```python
from build123d import *

# Parameters (mm, degrees)
SKETCH1_R           = 2
SKETCH1_R_2         = 4.5
BOSS_EXTRUDE1_DEPTH = 10
SKETCH1_3_R         = 4.5
BOSS_EXTRUDE2_DEPTH = 10
CUT_EXTRUDE1_DEPTH  = 13
FILLET1_R           = 1
FILLET2_R           = 1
SKETCH3_R           = 2.5
CUT_EXTRUDE2_DEPTH  = 10


with BuildPart() as part:
    # Sketch1 → Boss-Extrude1 (new body)
    with BuildSketch(Plane(origin=(0, 0, 0), x_dir=(1, 0, 0), z_dir=(0, 1, 0))):
        with BuildLine():
            ThreePointArc((-12, 5), (-11.707106781, 5.707106781), (-11, 6))
            Line((-11, 6), (11, 6))
            ThreePointArc((11, 6), (11.707106781, 5.707106781), (12, 5))
            Line((12, 5), (12, -5))
            ThreePointArc((12, -5), (11.707106781, -5.707106781), (11, -6))
            Line((11, -6), (-11, -6))
            ThreePointArc((-11, -6), (-11.707106781, -5.707106781), (-12, -5))
            Line((-12, -5), (-12, 5))
        make_face()
        with Locations((-8, 0)):
            Circle(SKETCH1_R, mode=Mode.SUBTRACT)
        with Locations((8, 0)):
            Circle(SKETCH1_R, mode=Mode.SUBTRACT)
        Circle(SKETCH1_R_2, mode=Mode.SUBTRACT)
        Circle(SKETCH1_R_2)
    extrude(amount=BOSS_EXTRUDE1_DEPTH)

    # Sketch1_3 → Boss-Extrude2 (add)
    with BuildSketch(Plane(origin=(0, 0, 0), x_dir=(1, 0, 0), z_dir=(0, 1, 0))):
        Circle(SKETCH1_3_R)
    extrude(amount=-BOSS_EXTRUDE2_DEPTH)

    # Sketch2 → Cut-Extrude1 (cut, through all)
    with BuildSketch(Plane.XY.offset(6)):
        with BuildLine():
            Line((-5, 10), (5, 10))
            ThreePointArc((5, 10), (0, 5), (-5, 10))
        make_face()
    extrude(amount=-CUT_EXTRUDE1_DEPTH, mode=Mode.SUBTRACT)

    # Fillet1
    fillet1_edges = [part.edges().sort_by_distance(p)[0] for p in [
        (0, 0, -6),
        (11.707106781, 0, -5.707106781),
        (12, 0, 0),
        (11.707106781, 0, 5.707106781),
        (0, 0, 6),
        (-11.707106781, 0, 5.707106781),
        (-12, 0, 0),
        (-11.707106781, 0, -5.707106781),
        (-4.5, -10, 0),
    ]]
    fillet(fillet1_edges, radius=FILLET1_R)

    # Fillet2
    fillet2_edges = [part.edges().sort_by_distance(p)[0] for p in [
        (-4.5, 0, 0),
    ]]
    fillet(fillet2_edges, radius=FILLET2_R)

    # Sketch3 → Cut-Extrude2 (cut)
    with BuildSketch(Plane.XZ.offset(10)):
        Circle(SKETCH3_R)
    extrude(amount=-CUT_EXTRUDE2_DEPTH, mode=Mode.SUBTRACT)


solid = part.part
```
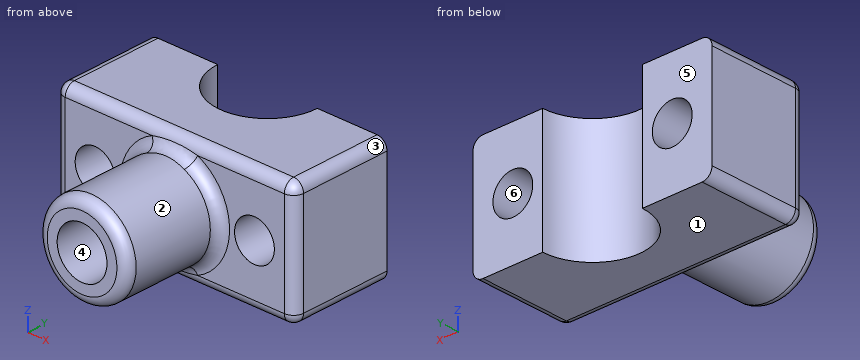
Geometry check sheet. Reference: the model listing, model coordinates, mm. Face numbers are marked on the shaded views. A direction names the side the tool comes from. Coordinates: 2 decimals unless noted, no trailing zeros. Loops run counter-clockwise (first coordinate to the right, second up) from the corner with the lowest first, then second, coordinate; pieces in that order, holes last.
Item 1: Sectioned sample at B-B, the plane y = 3.25. Record the boundary of the cut face in (x, z), then the cut area to 3 significant figures.
Item 2: Go/stop test with flat-tipped pins: pin 1 Ø2.5 at (x, z) = (-8, 0) entering from -Y; pin 2 Ø3 at (x, y) = (5.5, -4) entering from +Z; pin 3 Ø3 at (y, z) = (-4, -3.5) entering from +X; pin 4 Ø6 at (x, z) = (-6, 3) entering from -Y. Record where each tip stops, or that it passes through.
Item 3: Sectioned sample at C-C, the plane x = -8. Record the boundary of the cut face in (y, z).
Item 4: Access from +Z, -Z, +X, -X, +Y, -Y to the whole of each face (thin tool, end or side, straight path). Record for the marked faces 1 and 2.
Item 5: Sectioned sample at A-A, the plane y = 6. Record the boundary of the cut face in (x, z).
Item 6: Sectioned sample at D-D, the plane z = 0. Record the boundary of the cut face in (x, y).
Item 7: Release check for a two-part mould opening along Z. For the marked faces 3, 4, 5 and 6 record: released by +Z, released by -Z, zero draft, split by the parting line, or undercut.
Item 8: Thickness scan on line 1 (X direction, y = 2.25, z = 0); line 2 (Z direction, x = 8, y = 6.75); line 3 (X direction, y = 3, z = 1). Record the ranges inside material, lowest first.
Check result:
1. outline: (-12, -5) arc R1 ccw to (-11, -6) - (11, -6) arc R1 ccw to (12, -5) - (12, 5) arc R1 ccw to (11, 6) - (-11, 6) arc R1 ccw to (-12, 5) - close; hole circle Ø4 at (-8, 0); hole circle Ø4 at (8, 0)
1. area: 262 mm2
2. pin 1: passes through
2. pin 2: stops at z = 2.06
2. pin 3: stops at x = 4.03
2. pin 4: stops at y = -9.98
3. outline: (0, -5) arc R1 ccw to (1, -6) - (10, -6) - (10, -2) - (0, -2) - close; (0, 2) - (10, 2) - (10, 6) - (1, 6) arc R1 ccw to (0, 5) - close
4. face 1: -Z, +X, -X, +Y, -Y
4. face 2: -Y
5. outline: (-12, -5) arc R1 ccw to (-11, -6) - (-3, -6) - (-3, 6) - (-11, 6) arc R1 ccw to (-12, 5) - close; (3, -6) - (11, -6) arc R1 ccw to (12, -5) - (12, 5) arc R1 ccw to (11, 6) - (3, 6) - close; hole circle Ø4 at (-8, 0); hole circle Ø4 at (8, 0)
6. outline: (-12, 1) arc R1 ccw to (-11, 0) - (-10, 0) - (-10, 10) - (-12, 10) - close; (-6, 0) - (-5.5, 0) arc R1 cw to (-4.5, -1) - (-4.5, -9) arc R1 ccw to (-3.5, -10) - (-2.5, -10) - (-2.5, 0) - (2.5, 0) - (2.5, -10) - (3.5, -10) arc R1 ccw to (4.5, -9) - (4.5, -1) arc R1 cw to (5.5, 0) - (6, 0) - (6, 10) - (5, 10) arc R5 cw to (-5, 10) - (-6, 10) - close; (10, 0) - (11, 0) arc R1 ccw to (12, 1) - (12, 10) - (10, 10) - close
7. face 3: released by +Z
7. face 4: undercut
7. face 5: zero draft
7. face 6: undercut
8. line 1: x = -12 to -10, -6 to 6, 10 to 12
8. line 2: z = -6 to -2, 2 to 6
8. line 3: x = -12 to -9.73, -6.27 to 6.27, 9.73 to 12
